```python
from build123d import *

# Parameters (mm, degrees)
SKETCH1_R              = 4.7625
BODY_DEPTH             = 31.75
SKETCH3_R              = 18.288
PINION_CARRIER_DEPTH   = 44.45
SKETCH4_R              = 7.8994
PINION_DEPTH           = 64.3636
SKETCH5_R              = 12.7
PINION_BOTTOM_DEPTH    = 5.8674
PINION_BOTTOM_FILLET_R = 3.81
SKETCH2_R              = 10.31875
RACK_HOLE_DEPTH        = 51.8


with BuildPart() as part:
    # Sketch1 → Body (new body)
    with BuildSketch(Plane(origin=(0, 0, 0), x_dir=(1, 0, 0), z_dir=(0, 1, 0))):
        with BuildLine():
            Line((-7.493, -32.512), (7.493, -32.512))
            Line((7.493, -32.512), (8.032785528, -35.913455304))
            ThreePointArc((8.032785528, -35.913455304), (17.349253096, -43.254561784), (25.4, -34.544))
            Line((25.4, -34.544), (25.4, 0))
            Line((25.4, 0), (13.16736, 12.691397663))
            ThreePointArc((13.16736, 12.691397663), (0, 18.288), (-13.16736, 12.691397663))
            Line((-13.16736, 12.691397663), (-25.4, 0))
            Line((-25.4, 0), (-25.4, -34.544))
            ThreePointArc((-25.4, -34.544), (-17.349253096, -43.254561784), (-8.032785528, -35.913455304))
            Line((-8.032785528, -35.913455304), (-7.493, -32.512))
        make_face()
        with Locations((16.6624, -34.544)):
            Circle(SKETCH1_R, mode=Mode.SUBTRACT)
        with Locations((-16.6624, -34.544)):
            Circle(SKETCH1_R, mode=Mode.SUBTRACT)
    extrude(amount=BODY_DEPTH)

    # Sketch3 → Pinion Carrier (add)
    with BuildSketch(Plane.XZ):
        Circle(SKETCH3_R)
    extrude(amount=-PINION_CARRIER_DEPTH)

    # Sketch4 → Pinion (add)
    with BuildSketch(Plane.XZ):
        Circle(SKETCH4_R)
    extrude(amount=-PINION_DEPTH)

    # Sketch5 → Pinion Bottom (add)
    with BuildSketch(Plane.XZ):
        Circle(SKETCH5_R)
    extrude(amount=PINION_BOTTOM_DEPTH)

    # Pinion Bottom Fillet
    pinion_bottom_fillet_edges = [part.edges().sort_by_distance(p)[0] for p in [
        (-12.7, -5.8674, 0),
    ]]
    fillet(pinion_bottom_fillet_edges, radius=PINION_BOTTOM_FILLET_R)

    # Sketch2 → Rack Hole (cut, through all)
    with BuildSketch(Plane.ZY.offset(25.4)):
        with Locations((17.272, 15.875)):
            Circle(SKETCH2_R)
    extrude(amount=-RACK_HOLE_DEPTH, mode=Mode.SUBTRACT)


solid = part.part
```
For this review, take the finished solid that the model builds, in its own axes (mm). A direction names the side the tool comes from. Coordinates: 2 decimals unless noted, no trailing zeros. Loops run counter-clockwise (first coordinate to the right, second up) from the corner with the lowest first, then second, coordinate; pieces in that order, holes last. Notation, with made-up numbers: (-36, 3) -> (-32, 3) arc R25 ccw to (-32, 16) -> close; hole circle Ø9 at (63, 3.5). An arc over 180 degrees is marked (long way). Return JSON: item names as keys, results as strings. Group by question number.
(1) Consider section A-A, the plane y = 11. Give the boundary of the cut face in (x, z) (1 decimal).
(2) Tool access review of faces 4 (the flat face through (-7.767, 15.653, 34.237)), 5 (the cylindrical face through (-12.12, 15.65, 33.11)), 6 (the flat face through (8, 44.45, -4)): name each direction out of +Z, -Z, +X, -X, +Y, -Y from which nothing blocks a thin tool from reaching the whole face with its end or side.
(3) For pin 1 Ø1 at (x, y) = (-20, 26.5) entering from -Z; pin 2 Ø4 at (x, y) = (-14.5, 47) entering from +Z; pin 3 Ø8 at (x, z) = (-18.5, 17.5) entering from +Y; pin 4 Ø5 at (x, z) = (-13.5, 24.5) entering from -Y, all flat-tipped, find the tip position at first contact; note any pin that passes through.
(4) Consider section D-D, the plane z = 38. Give the boundary of the cut face in (x, y), plus the area to 3 significant figures.
(5) Consider section B-B, the plane x = -16. Count the separate pieces of the cut face and the enclosed holes in it, plus the area to 3 significant figures.
(6) Mouldability with a two-part tool opening along X and no side actions: class faces 1 (the cylindrical face through (-2.75, -1.01, -12.4)), 2 (the flat face through (0, 31.75, 21)), 3 (the flat face through (7.76, 15.65, 34.19)) as pulls with the +X half, pulls with the -X half, needs draft (parallel to the pull), parting line crosses it, or undercut.
(7) To check wall thickness, follow L1, parallel to Y at x = -17.5, z = 22; L2, parallel to Z at x = -11, y = 13; L3, parallel to Y at x = 23, z = 40.5. State the ranges of each line that lie inside material, in increasing order.
(8) Consider section C-C, the plane y = 29. Give the boundary of the cut face in (x, z) (1 decimal), plus the area to 3 significant figures.
Results below:
{
 "1": {"outline": "(-25.4, 0) -> (-13.2, -12.7) arc R18.3 ccw to (13.2, -12.7) -> (25.4, 0) -> (25.4, 8.2) -> (-25.4, 8.2) -> close; (-25.4, 26.4) -> (25.4, 26.4) -> (25.4, 34.5) arc R8.7 ccw to (8, 35.9) -> (7.5, 32.5) -> (-7.5, 32.5) -> (-8, 35.9) arc R8.7 ccw to (-25.4, 34.5) -> close; hole circle Ø9.5 at (-16.7, 34.5); hole circle Ø9.5 at (16.7, 34.5)"},
 "2": {"face 4": "+Z, +Y, -Y", "face 5": "+Y, -Y", "face 6": "+Y"},
 "3": {"pin 1": "stops at z = -6.12", "pin 2": "passes through", "pin 3": "stops at y = 31.75", "pin 4": "stops at y = 0"},
 "4": {"outline": "(-24.69, 0) -> (-19.94, 0) -> (-19.94, 31.75) -> (-24.69, 31.75) -> close; (-13.39, 0) -> (-8.64, 0) -> (-8.64, 31.75) -> (-13.39, 31.75) -> close; (8.64, 0) -> (13.39, 0) -> (13.39, 31.75) -> (8.64, 31.75) -> close; (19.94, 0) -> (24.69, 0) -> (24.69, 31.75) -> (19.94, 31.75) -> close", "area": "603 mm2"},
 "5": {"separate pieces": "2", "enclosed holes": "1", "area": "1,270 mm2"},
 "6": {"face 1": "parting line crosses it", "face 2": "needs draft", "face 3": "undercut"},
 "7": {"L1": "y = 0 to 6.7, 25.05 to 31.75", "L2": "z = -14.61 to 7.36, 27.18 to 41.2", "L3": "y = 0 to 31.75"},
 "8": {"outline": "(-25.4, 0) -> (-13.2, -12.7) arc R18.3 ccw to (13.2, -12.7) -> (25.4, 0) -> (25.4, 34.5) arc R8.7 ccw to (8, 35.9) -> (7.5, 32.5) -> (-7.5, 32.5) -> (-8, 35.9) arc R8.7 ccw to (-25.4, 34.5) -> close; hole circle Ø9.5 at (-16.7, 34.5); hole circle Ø9.5 at (16.7, 34.5)", "area": "2,410 mm2"}
}
